```python
from build123d import *

# Parameters (mm, degrees)
SKETCH1_R            = 80
BOSS_EXTRUDE1_DEPTH  = 16
SKETCH2_R            = 22.5
BOSS_EXTRUDE2_DEPTH  = 62
BOSS_EXTRUDE3_DEPTH  = 22
SKETCH4_R            = 22.5
BOSS_EXTRUDE4_DEPTH  = 35
BOSS_EXTRUDE5_DEPTH  = 25
SKETCH6_R            = 22.5
BOSS_EXTRUDE6_DEPTH  = 35
BOSS_EXTRUDE7_DEPTH  = 22
SKETCH8_R            = 25
BOSS_EXTRUDE8_DEPTH  = 45
BOSS_EXTRUDE9_DEPTH  = 22
SKETCH10_R           = 22.5
BOSS_EXTRUDE10_DEPTH = 22
BOSS_EXTRUDE11_DEPTH = 25
SKETCH12_R           = 22.5
BOSS_EXTRUDE12_DEPTH = 35
BOSS_EXTRUDE13_DEPTH = 22
SKETCH14_R           = 22.5
BOSS_EXTRUDE14_DEPTH = 45
SKETCH15_R           = 25
BOSS_EXTRUDE15_DEPTH = 100
SKETCH16_R           = 12.5
BOSS_EXTRUDE16_DEPTH = 20
SKETCH17_R           = 6
CUT_EXTRUDE1_DEPTH   = 16
CIRPATTERN1_COUNT    = 4


with BuildPart() as part:
    # Sketch1 → Boss-Extrude1 (new body)
    with BuildSketch(Plane.XY):
        Circle(SKETCH1_R)
    extrude(amount=BOSS_EXTRUDE1_DEPTH)

    # Sketch2 → Boss-Extrude2 (add)
    with BuildSketch(Plane.XY.offset(16)):
        Circle(SKETCH2_R)
    extrude(amount=BOSS_EXTRUDE2_DEPTH)

    # Sketch3 → Boss-Extrude3 (add)
    with BuildSketch(Plane.XY.offset(78)):
        with BuildLine():
            Line((0, -27.5), (-40, -27.5))
            ThreePointArc((-40, -27.5), (-67.5, 0), (-40, 27.5))
            Line((-40, 27.5), (0, 27.5))
            ThreePointArc((0, 27.5), (27.5, 0), (0, -27.5))
        make_face()
    extrude(amount=BOSS_EXTRUDE3_DEPTH)

    # Sketch4 → Boss-Extrude4 (add)
    with BuildSketch(Plane.XY.offset(100)):
        with Locations((-40, 0)):
            Circle(SKETCH4_R)
    extrude(amount=BOSS_EXTRUDE4_DEPTH)

    # Sketch5 → Boss-Extrude5 (add)
    with BuildSketch(Plane.XY.offset(135)):
        with BuildLine():
            Line((-40, 27.5), (40, 27.5))
            ThreePointArc((40, 27.5), (67.5, 0), (40, -27.5))
            Line((40, -27.5), (-40, -27.5))
            ThreePointArc((-40, -27.5), (-67.5, 0), (-40, 27.5))
        make_face()
    extrude(amount=BOSS_EXTRUDE5_DEPTH)

    # Sketch6 → Boss-Extrude6 (add)
    with BuildSketch(Plane.XY.offset(160)):
        with Locations((40, 0)):
            Circle(SKETCH6_R)
    extrude(amount=BOSS_EXTRUDE6_DEPTH)

    # Sketch7 → Boss-Extrude7 (add)
    with BuildSketch(Plane.XY.offset(195)):
        with BuildLine():
            Line((40, -27.5), (0, -27.5))
            ThreePointArc((0, -27.5), (-27.5, 0), (0, 27.5))
            Line((0, 27.5), (40, 27.5))
            ThreePointArc((40, 27.5), (67.5, 0), (40, -27.5))
        make_face()
    extrude(amount=BOSS_EXTRUDE7_DEPTH)

    # Sketch8 → Boss-Extrude8 (add)
    with BuildSketch(Plane.XY.offset(217)):
        Circle(SKETCH8_R)
    extrude(amount=BOSS_EXTRUDE8_DEPTH)

    # Sketch9 → Boss-Extrude9 (add)
    with BuildSketch(Plane.XY.offset(262)):
        with BuildLine():
            Line((40, 27.5), (0, 27.5))
            ThreePointArc((0, 27.5), (-27.5, 0), (0, -27.5))
            Line((0, -27.5), (40, -27.5))
            ThreePointArc((40, -27.5), (67.5, 0), (40, 27.5))
        make_face()
    extrude(amount=BOSS_EXTRUDE9_DEPTH)

    # Sketch10 → Boss-Extrude10 (add)
    with BuildSketch(Plane.XY.offset(284)):
        with Locations((40, 0)):
            Circle(SKETCH10_R)
    extrude(amount=BOSS_EXTRUDE10_DEPTH)

    # Sketch11 → Boss-Extrude11 (add)
    with BuildSketch(Plane.XY.offset(306)):
        with BuildLine():
            Line((40, -27.5), (-40, -27.5))
            ThreePointArc((-40, -27.5), (-67.5, 0), (-40, 27.5))
            Line((-40, 27.5), (40, 27.5))
            ThreePointArc((40, 27.5), (67.5, 0), (40, -27.5))
        make_face()
    extrude(amount=BOSS_EXTRUDE11_DEPTH)

    # Sketch12 → Boss-Extrude12 (add)
    with BuildSketch(Plane.XY.offset(331)):
        with Locations((-40, 0)):
            Circle(SKETCH12_R)
    extrude(amount=BOSS_EXTRUDE12_DEPTH)

    # Sketch13 → Boss-Extrude13 (add)
    with BuildSketch(Plane.XY.offset(366)):
        with BuildLine():
            Line((-40, 27.5), (0, 27.5))
            ThreePointArc((0, 27.5), (27.5, 0), (0, -27.5))
            Line((0, -27.5), (-40, -27.5))
            ThreePointArc((-40, -27.5), (-67.5, 0), (-40, 27.5))
        make_face()
    extrude(amount=BOSS_EXTRUDE13_DEPTH)

    # Sketch14 → Boss-Extrude14 (add)
    with BuildSketch(Plane.XY.offset(388)):
        Circle(SKETCH14_R)
    extrude(amount=BOSS_EXTRUDE14_DEPTH)

    # Sketch15 → Boss-Extrude15 (add)
    with BuildSketch(Plane.XY.offset(433)):
        Circle(SKETCH15_R)
    extrude(amount=BOSS_EXTRUDE15_DEPTH)

    # Sketch16 → Boss-Extrude16 (add)
    with BuildSketch(Plane.XY.offset(533)):
        Circle(SKETCH16_R)
    extrude(amount=BOSS_EXTRUDE16_DEPTH)

    # Sketch17 → Cut-Extrude1 (cut)
    with BuildSketch(Plane(origin=(0, 0, 0), x_dir=(-1, 0, 0), z_dir=(0, 0, -1))):
        with Locations((0, 40)):
            Circle(SKETCH17_R)
    cut_extrude1 = extrude(amount=-CUT_EXTRUDE1_DEPTH, mode=Mode.SUBTRACT)

    # CirPattern1: Cut-Extrude1 ×4 about axis
    cirpattern1_axis = Axis((0, 0, 0), (0, 0, 1))
    for i in range(1, CIRPATTERN1_COUNT):
        add(cut_extrude1.rotate(cirpattern1_axis, i * 360 / CIRPATTERN1_COUNT), mode=Mode.SUBTRACT)


solid = part.part
```
Geometry check sheet. Reference: the model listing, model coordinates, mm. A direction names the side the tool comes from. Round coordinates to 2 decimals unless told otherwise and drop trailing zeros. Order: outer loops, then holes, each group sorted by start corner. A loop starts at its lowest first (then second) coordinate and runs counter-clockwise, first axis right, second up. Notation, with made-up numbers: M 63,-17.75 L 102,-17.75 A37 ccw 102,21.25 Z; hole C 25.5,14.5 d5. An arc over 180 degrees is marked long. Answer as CSV lines item,"result".
1) Sectioned sample at D-D on z = 481. Record the cut outline in (x, y), and give its area (3 significant figures).
Entries:
outline,"C 0,0 d50"
area,"1,960 mm2"
2) Thickness scan on probe 1 along Y at (x, z) = (0, 4.25); probe 2 along Z at (x, y) = (-7.5, 29); probe 3 along Y at (x, z) = (-40, 10). Record the ranges inside material, lowest first. Write a range as [from, to].
Entries:
probe 1,"[-80, -46], [-34, 34], [46, 80]"
probe 2,"[0, 16]"
probe 3,"[-69.28, -6], [6, 69.28]"
3) Mould release check, pull along Z, two halves, no side actions. Record for faces 1 (the face through (27.493, 0.605, 88.846)), 2 (the face through (-20, 27.5, 377)): +Z half, -Z half, draft (parallel to the pull), parting line (faces both ways), or undercut.
Entries:
face 1,"undercut"
face 2,"draft"
4) Tool access check on faces 3 (the face through (-27.493, 0.605, 272.846)), 4 (the face through (22.145, -13.691, 177.255)), 5 (the face through (23.846, 7.509, 482.3)), 6 (the face through (-20, 27.5, 89)), 7 (the face through (34.143, -1.301, 7.888)). Record the directions out of +Z, -Z, +X, -X, +Y, -Y that give a thin tool (end or side, any length) a straight path to the whole face; none if there is none.
Entries:
face 3,"-X"
face 4,"none"
face 5,"+Z"
face 6,"+Z, +X, -X, +Y"
face 7,"-Z"
5) Sectioned sample at C-C on z = 403. Record the cut outline in (x, y), and give its area (3 significant figures).
Entries:
outline,"C 0,0 d45"
area,"1,590 mm2"
6) Gauge pin test, flat ends, axial feed: pin 1 Ø5 at (y, z) = (7.5, 444.5) entering from -X; pin 2 Ø11 at (x, z) = (21.5, 274.5) entering from +Y; pin 3 Ø4 at (x, z) = (61.5, 281.5) entering from -Y. Record the tip position at first contact, or that the pin passes through.
Entries:
pin 1,"x = -24.49"
pin 2,"y = 27.5"
pin 3,"y = -19.39"
7) Sectioned sample at A-A on y = 40. Record the cut outline in (x, z).
Entries:
outline,"M -69.28,0 L -6,0 L -6,16 L -69.28,16 Z; M 6,0 L 69.28,0 L 69.28,16 L 6,16 Z"
8) Sectioned sample at B-B on z = 209. Record the cut outline in (x, y), and give its area (3 significant figures).
Entries:
outline,"M 0,-27.5 L 40,-27.5 A27.5 ccw 40,27.5 L 0,27.5 A27.5 ccw Z"
area,"4,580 mm2"
